Part model, mm, in its own coordinate system. Face numbers are marked on the shaded views. A direction names the side the tool comes from. Give positions to 0.01 mm unless a question says otherwise; leave off trailing zeros. Loops run counter-clockwise (first coordinate to the right, second up) from the corner with the lowest first, then second, coordinate; pieces in that order, holes last. Notation, with made-up numbers: (-14.5, -13) -> (24.5, -13) arc R15 ccw to (24.5, 2) -> close; hole circle Ø11 at (4, -28.5). An arc over 180 degrees is marked (long way). Write item = value, one per line.
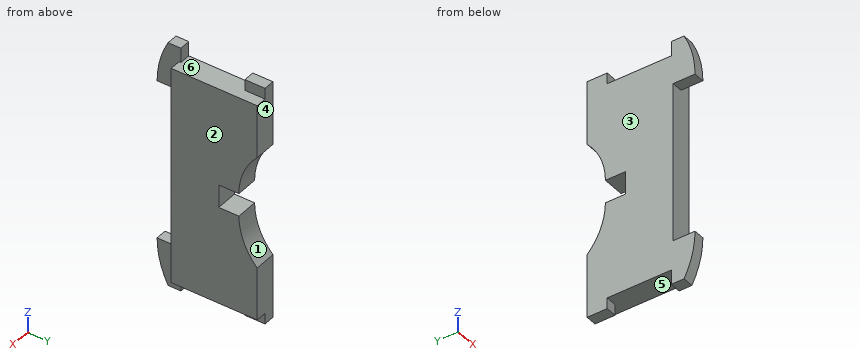
from build123d import *

# Parameters (mm, degrees)
BOSS_EXTRUDE1_DEPTH = 3
BOSS_EXTRUDE2_START = 3
BOSS_EXTRUDE2_DEPTH = 3


with BuildPart() as part:
    # Sketch1 → Boss-Extrude1 (new body)
    with BuildSketch(Plane(origin=(0, 0, 0), x_dir=(0, 0, -1), z_dir=(1, 0, 0))):
        with BuildLine():
            Line((-3.15, 0), (3.15, 0))
            Line((3.15, 0), (3.15, 5.5))
            ThreePointArc((3.15, 5.5), (9.788712225, 6.797767928), (15.45, 10.5))
            Line((15.45, 10.5), (30, 10.5))
            Line((30, 10.5), (30, -13))
            Line((30, -13), (-30, -13))
            Line((-30, -13), (-30, 10.5))
            Line((-30, 10.5), (-15.45, 10.5))
            ThreePointArc((-15.45, 10.5), (-9.788712225, 6.797767928), (-3.15, 5.5))
            Line((-3.15, 5.5), (-3.15, 0))
        make_face()
    extrude(amount=BOSS_EXTRUDE1_DEPTH)

    # Sketch2 → Boss-Extrude2 (add)
    with BuildSketch(Plane.ZY.offset(BOSS_EXTRUDE2_START)):
        with BuildLine():
            Line((34, -12.5), (30, -12.5))
            Line((30, -12.5), (30, 5))
            Line((30, 5), (33, 5))
            Line((33, 5), (33, 10.5))
            Line((33, 10.5), (15.45, 10.5))
            ThreePointArc((15.45, 10.5), (9.788712225, 6.797767928), (3.15, 5.5))
            Line((3.15, 5.5), (3.15, 0))
            Line((3.15, 0), (-3.15, 0))
            Line((-3.15, 0), (-3.15, 5.5))
            ThreePointArc((-3.15, 5.5), (-9.788712225, 6.797767928), (-15.45, 10.5))
            Line((-15.45, 10.5), (-33, 10.5))
            Line((-33, 10.5), (-33, 5))
            Line((-33, 5), (-30, 5))
            Line((-30, 5), (-30, -12.5))
            Line((-30, -12.5), (-34, -12.5))
            Line((-34, -12.5), (-34, -16))
            ThreePointArc((-34, -16), (-28.184658438, -18.238633754), (-22, -19))
            Line((-22, -19), (-22, -13))
            Line((-22, -13), (22, -13))
            Line((22, -13), (22, -19))
            ThreePointArc((22, -19), (28.184658438, -18.238633754), (34, -16))
            Line((34, -16), (34, -12.5))
        make_face()
    extrude(amount=-BOSS_EXTRUDE2_DEPTH)


solid = part.part
1) Which spindle directions (+Z, -Z, +X, -X, +Y, -Y) get a long thin tool onto all of the face, cutting with end or side? Do the marked faces 1 and 2. Say none if no direction does.
Resolved:
face_1 = +X, -X, +Y
face_2 = +Z, -Z, +X, +Y, -Y
2) Drop flat-ended pins along their axis: P1, Ø2, axis at x = -2, y = -5, coming from the -Z side; P2, Ø3.5, axis at x = -1, y = 8, coming from the -Z side; P3, Ø3, axis at y = -15.5, z = 26.5, coming from the +X side. Give the stop position or say it passes through.
Resolved:
P1 = -30
P2 = -33
P3 = 0
3) Slice it at A-A, the plane y = -14.25. List the corners of the cut face in (x, z).
Resolved:
outline = (-3, -34) -> (0, -34) -> (0, -22) -> (-3, -22) -> close; (-3, 22) -> (0, 22) -> (0, 34) -> (-3, 34) -> close
4) Slice it at B-B, the plane x = 1.2. List the corners of the cut face in (y, z).
Resolved:
outline = (-13, -30) -> (10.5, -30) -> (10.5, -15.45) arc R17.63 cw to (5.5, -3.15) -> (0, -3.15) -> (0, 3.15) -> (5.5, 3.15) arc R17.63 cw to (10.5, 15.45) -> (10.5, 30) -> (-13, 30) -> close
5) Pull direction Y, two halves, no side cores. Call the marked faces 3, 4, 5 and 6: pulls with the +Y half, pulls with the -Y half, needs draft (parallel to the pull), parting line crosses it, or undercut.
Resolved:
face_3 = needs draft
face_4 = pulls with the +Y half
face_5 = undercut
face_6 = undercut
6) Slice it at C-C, the plane z = 1. List the corners of the cut face in (x, y), and give its area (3 significant figures).
Resolved:
outline = (-3, -13) -> (3, -13) -> (3, 0) -> (-3, 0) -> close
area = 78.0 mm²
7) Drill centre lines: line 1 along Z through (x, y) = (-1.4, 4); line 2 along Y through (x, z) = (-1.3, -1.5); line 3 along Z through (x, y) = (-1.8, -9). Where is each one in solid material? Low to high. Write a range as [from, to].
Resolved:
line_1 = [-30, -3.15], [3.15, 30]
line_2 = [-13, 0]
line_3 = [-30, 30]
8) Slice it at D-D, the plane x = -2.4. List the corners of the cut face in (y, z).
Resolved:
outline = (-19, -22) arc R25.5 ccw to (-16, -34) -> (-12.5, -34) -> (-12.5, -30) -> (5, -30) -> (5, -33) -> (10.5, -33) -> (10.5, -15.45) arc R17.63 cw to (5.5, -3.15) -> (0, -3.15) -> (0, 3.15) -> (5.5, 3.15) arc R17.63 cw to (10.5, 15.45) -> (10.5, 33) -> (5, 33) -> (5, 30) -> (-12.5, 30) -> (-12.5, 34) -> (-16, 34) arc R25.5 ccw to (-19, 22) -> (-13, 22) -> (-13, -22) -> close
